Work out the finished part from the listing and answer in its coordinate system (mm). A direction names the side the tool comes from. Coordinates: 2 decimals unless noted, no trailing zeros. Write each loop counter-clockwise with the first axis right and the second up, starting at its lowest first coordinate (ties: lowest second). Pieces come first, ordered by that corner, then holes. Notation, with made-up numbers: M 42,-40 L 94,-40 A9 ccw 94,-26 Z; hole C 47.5,23 d4. An arc over 180 degrees is marked long. Answer as CSV lines item,"result". Start each with the question number.
(1) A cutting plane is placed at B-B on z = 0. Give the vertices of the cut face in (x, y).
(2) Find the intervals of material crossed by L1, parallel to Y at x = 2.5, z = -5.5; L2, parallel to Y at x = 0, z = -2.75; L3, parallel to Z at x = 0.5, y = -9, in increasing order. Write a range as [from, to].
(3) A cutting plane is placed at D-D on x = 6.75. Give the vertices of the cut face in (y, z), then the cut area to 3 significant figures.
(4) A cutting plane is placed at A-A on x = 0. Give the vertices of the cut face in (y, z).
(5) A cutting plane is placed at C-C on y = 15.5. Give the vertices of the cut face in (x, z), then the cut area to 3 significant figures.
(6) For faces 1 (the cylindrical face through (0.647, 14.689, 2.914)), 2 (the flat face through (0, 24, -1.46)), 3 (the flat face through (0, 29.794, 0)), determine the directions among +Z, -Z, +X, -X, +Y, -Y from which every point of the face is accessible in a straight line to the end or side of a thin tool.
(7) Flat-ended cylindrical pins translate along their axes: P1, Ø4, axis at x = -1, y = 17.5, coming from the +Z side; P2, Ø5, axis at y = 25, z = 0, coming from the -X side; P3, Ø5, axis at y = 1.5, z = 6.5, coming from the -X side. Find the tip coordinate at first contact, or state that the pin passes through.
Autodesk Inventor part; units mm, degrees
ref_plane "YZ Plane" through (0, 0, 0) normal (1, 0, 0) x (0, 1, 0)
ref_plane "XZ Plane" through (0, 0, 0) normal (0, 1, 0) x (-1, 0, 0)
ref_plane "XY Plane" through (0, 0, 0) normal (0, 0, 1) x (1, 0, 0)
sketch "Sketch1" plane through (0, 0, 0) normal (0, 1, 0) x (-1, 0, 0)
  circle A0 centre (0, 0) radius 8.382
  circle A1 centre (0, 0) radius 2.9845
  dimension "d0" = 5.969
  dimension "d1" = 16.764
extrude "Extrusion1" add sketch "Sketch1" against normal blind 11.176 contours A0 | A1
extrude "Extrusion2" add sketch "Sketch1" along normal blind 29.7942 contours A1
sketch "Sketch2" plane through (0, 29.7942, 0) normal (0, 1, 0) x (1, 0, 0)
  circle A0 centre (0, 0) radius 2.9845
  circle A1 centre (0, 0) radius 2.9845
  line L0 (-2.6027, 1.4605) -> (2.6027, 1.4605)
  arc A2 (2.6027, 1.4605) -> (-2.6027, 1.4605) centre (0, 0) ccw
  dimension "d6" = 4.445
extrude "Extrusion3" cut sketch "Sketch2" against normal blind 11.8872 contours L0 A0 picked at (-0.1168, 1.9616)
properties part number "Potentiometer"
Here are the results:
1,outline,"M -8.38,-11.18 L 8.38,-11.18 L 8.38,0 L 2.98,0 L 2.98,29.79 L -2.98,29.79 L -2.98,0 L -8.38,0 Z"
2,L1,"y = [-11.18, 0]"
2,L2,"y = [-11.18, 17.91]"
2,L3,"z = [-8.37, 8.37]"
3,outline,"M -11.18,-4.97 L 0,-4.97 L 0,4.97 L -11.18,4.97 Z"
3,area,"111 mm^2"
4,outline,"M -11.18,-8.38 L 0,-8.38 L 0,-2.98 L 17.91,-2.98 L 17.91,-1.46 L 29.79,-1.46 L 29.79,2.98 L 0,2.98 L 0,8.38 L -11.18,8.38 Z"
5,outline,"C 0,0 d5.97"
5,area,"28.0 mm^2"
6,face 1,"+Y"
6,face 2,"-Z, +X, -X, +Y"
6,face 3,"+Z, -Z, +X, -X, +Y"
7,P1,"stops at z = 2.98"
7,P2,"stops at x = -2.98"
7,P3,"stops at x = -7.07"
